Input: part model. Units: mm. Frame: model coordinates. Face numbers are marked on the shaded views. A direction names the side the tool comes from. Coordinates: 2 decimals unless noted, no trailing zeros. Order: outer loops, then holes, each group sorted by start corner. A loop starts at its lowest first (then second) coordinate and runs counter-clockwise, first axis right, second up. Notation, with made-up numbers: (-5.5, 70.25) -> (35.5, 70.25) arc R32 ccw to (35.5, 109.25) -> close; hole circle Ø10 at (88.25, 64.5). An arc over 180 degrees is marked (long way). One line per question, with ' | ' between items.
```python
from build123d import *

# Parameters (mm, degrees)
BOSS_EXTRUDE1_DEPTH = 15
BOSS_EXTRUDE2_DEPTH = 15
CUT_EXTRUDE1_REACH  = 40.406
SKETCH2_R           = 1.75
CUT_EXTRUDE4_START  = -15
SKETCH5_W           = 78.790180628
SKETCH5_H           = 1
CUT_EXTRUDE4_DEPTH  = 15
SKETCH3_R           = 3.25
CUT_EXTRUDE2_DEPTH  = 9
FILLET1_R           = 3.5


with BuildPart() as part:
    # Sketch1 → Boss-Extrude1 (new body)
    with BuildSketch(Plane(origin=(0, 0, 0), x_dir=(1, 0, 0), z_dir=(0, 1, 0))):
        with BuildLine():
            Line((-6.6, 0), (-14.6, 0))
            ThreePointArc((-14.6, 0), (0, 14.6), (14.6, 0))
            Line((14.6, 0), (6.6, 0))
            ThreePointArc((6.6, 0), (0, 6.6), (-6.6, 0))
        make_face()
    extrude(amount=BOSS_EXTRUDE1_DEPTH)

    # Sketch6 → Boss-Extrude2 (add)
    with BuildSketch(Plane.XZ):
        with BuildLine():
            Line((-25, 0), (-8.641827511, 0))
            ThreePointArc((-8.641827511, 0), (0, -8.641827511), (8.641827511, 0))
            Line((8.641827511, 0), (25, 0))
            ThreePointArc((25, 0), (21.153421014, -7.882601717), (12.572918035, -9.70099341))
            ThreePointArc((12.572918035, -9.70099341), (11.366290804, -9.716055468), (10.323759005, -10.323759005))
            ThreePointArc((10.323759005, -10.323759005), (9.716055468, -11.366290804), (9.70099341, -12.572918035))
            ThreePointArc((9.70099341, -12.572918035), (0, -25), (-9.70099341, -12.572918035))
            ThreePointArc((-9.70099341, -12.572918035), (-9.716055468, -11.366290804), (-10.323759005, -10.323759005))
            ThreePointArc((-10.323759005, -10.323759005), (-11.366290804, -9.716055468), (-12.572918035, -9.70099341))
            ThreePointArc((-12.572918035, -9.70099341), (-21.153421014, -7.882601717), (-25, 0))
        make_face()
    extrude(amount=-BOSS_EXTRUDE2_DEPTH)

    # Sketch2 → Cut-Extrude1 (cut, up to next)
    with BuildSketch(Plane(origin=(0, 0, 0), x_dir=(-1, 0, 0), z_dir=(0, 0, -1)), mode=Mode.PRIVATE) as cut_extrude1_sk1:
        with Locations(Location((-13.6, 7.5, 0), (0, 0, 54.062388323))):
            Circle(SKETCH2_R)
    cut_extrude1_tool1 = extrude(cut_extrude1_sk1.sketch, amount=CUT_EXTRUDE1_REACH, mode=Mode.PRIVATE) & part.part
    # Sketch2 → Cut-Extrude1 (cut, up to next)
    with BuildSketch(Plane(origin=(0, 0, 0), x_dir=(-1, 0, 0), z_dir=(0, 0, -1)), mode=Mode.PRIVATE) as cut_extrude1_sk2:
        with Locations(Location((13.6, 7.5, 0), (0, 0, 234.062388323))):
            Circle(SKETCH2_R)
    cut_extrude1_tool2 = extrude(cut_extrude1_sk2.sketch, amount=CUT_EXTRUDE1_REACH, mode=Mode.PRIVATE) & part.part
    add(cut_extrude1_tool1.solids().sort_by_distance((13.6, 7.5, 0))[0], mode=Mode.SUBTRACT)
    add(cut_extrude1_tool2.solids().sort_by_distance((-13.6, 7.5, 0))[0], mode=Mode.SUBTRACT)

    # Sketch5 → Cut-Extrude4 (cut)
    with BuildSketch(Plane(origin=(0, 15, 0), x_dir=(1, 0, 0), z_dir=(0, 1, 0)).offset(CUT_EXTRUDE4_START)):
        with Locations((-1.565702307, 0.5)):
            Rectangle(SKETCH5_W, SKETCH5_H)
    extrude(amount=CUT_EXTRUDE4_DEPTH, mode=Mode.SUBTRACT)

    # Sketch3 → Cut-Extrude2 (cut)
    with BuildSketch(Plane.XY.offset(-15)):
        with Locations(Location((13.6, 7.5, 0), (0, 0, 180))):
            Circle(SKETCH3_R)
        Polygon((-10.8, 5.883419246), (-10.8, 9.116580754), (-13.6, 10.733161507), (-16.4, 9.116580754), (-16.4, 5.883419246), (-13.6, 4.266838493), align=None)
    extrude(amount=CUT_EXTRUDE2_DEPTH, mode=Mode.SUBTRACT)

    # Fillet1
    fillet1_edges = [part.edges().sort_by_distance(p)[0] for p in [
        (10.323759005, 0, -10.323759005),
        (20.751080157, 0, -8.180774843),
        (-10.323759005, 0, -10.323759005),
        (0, 0, -25),
        (10.323759005, 15, -10.323759005),
        (-10.323759005, 15, -10.323759005),
        (-20.751080157, 15, -8.180774843),
        (0, 15, -25),
        (-20.751080157, 0, -8.180774843),
        (20.751080157, 15, -8.180774843),
    ]]
    fillet(fillet1_edges, radius=FILLET1_R)


solid = part.part
```
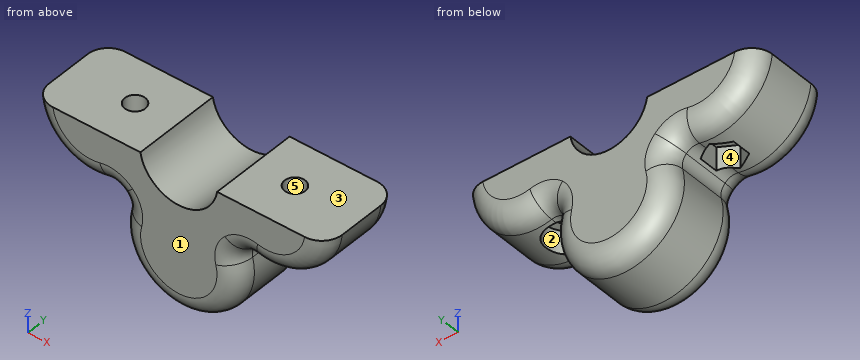
1. Ray query, line 1 (Y direction, x = 13.6, z = -2.15); line 2 (X direction, y = 7.5, z = -5); line 3 (X direction, y = 7.5, z = -7.8). Return the intervals inside material, ascending. Write a range as [from, to].
Recorded:
line 1: y = [0, 5.75], [9.25, 15] | line 2: x = [-23.66, -15.35], [-11.85, -4.31], [4.31, 11.85], [15.35, 23.66] | line 3: x = [-21.26, -16.4], [-10.8, 10.35], [16.85, 21.26]
2. Cut plane B-B, the plane x = 0. Return loops of the section in (y, z), and give its area (3 significant figures).
Recorded:
outline: (0, -21.5) arc R3.5 ccw to (3.5, -25) -> (11.5, -25) arc R3.5 ccw to (15, -21.5) -> (15, -6.6) -> (0, -6.6) -> close | area: 271 mm^2
3. Cut plane A-A, the plane y = 7.5. Return loops of the section in (x, z), and give its area (3 significant figures).
Recorded:
outline: (-24.95, -1) arc R10 ccw to (-16.4, -9.9) -> (-16.4, -6) -> (-15.35, -6) -> (-15.35, -1) -> close; (-11.85, -6) -> (-10.8, -6) -> (-10.8, -9.96) arc R2.37 cw to (-9.7, -12.57) arc R10 ccw (long way) to (9.7, -12.57) arc R2.37 cw to (10.35, -10.3) -> (10.35, -6) -> (11.85, -6) -> (11.85, -1) -> (6.52, -1) arc R6.6 cw to (-6.52, -1) -> (-11.85, -1) -> close; (15.35, -6) -> (16.85, -6) -> (16.85, -9.83) arc R10 ccw to (24.95, -1) -> (15.35, -1) -> close | area: 525 mm^2
4. Pin query (flat end, axial travel): pin 1 Ø1.7 at (x, y) = (-13, 6) entering from -Z; pin 2 Ø1.5 at (y, z) = (5, -12.5) entering from +X; pin 3 Ø2 at (y, z) = (4, -14.5) entering from -X. Return the tip coordinate at first contact, or that it passes through.
Recorded:
pin 1: stops at z = -6 | pin 2: stops at x = 9.85 | pin 3: stops at x = -10
5. Access query for the marked faces 4 and 5. Directions: +Z, -Z, +X, -X, +Y, -Y. A direction counts if a zero-diameter tool reaches every point of the face in a straight line with its end or side. Return the directions, or none.
Recorded:
face 4: -Z | face 5: +Z, -Z
6. Mould query, pull axis Y, two halves, no side actions, for the marked faces 1, 2 and 3. Classes: released by +Y, released by -Y, zero draft, split by the parting line, or undercut.
Recorded:
face 1: released by -Y | face 2: undercut | face 3: zero draft
